Read the model definition and answer for the solid it produces. Units are mm, in the model's axes. Face numbers are marked on the shaded views. A direction names the side the tool comes from. Round coordinates to 2 decimals unless told otherwise and drop trailing zeros. Order: outer loops, then holes, each group sorted by start corner. A loop starts at its lowest first (then second) coordinate and runs counter-clockwise, first axis right, second up. Notation, with made-up numbers: (-29, 65) - (26, 65) arc R24 cw to (26, 95) - close; hole circle Ø10 at (81.5, 83.5). An arc over 180 degrees is marked (long way). Put each result on its own line as item: value. Start each with the question number.
Q1. Each of these flat-tipped pins is pushed along its axis until it touches: pin 1 Ø22 at (x, y) = (8, -12.5) entering from +Z; pin 2 Ø3 at (x, z) = (-8.5, 17.5) entering from -Y; pin 3 Ø2.5 at (y, z) = (26.5, 17.5) entering from +X. Where does it stop, or does it pass through?
Q2. Section C-C on x = 16 is taken. Give the vertices of the cut face in (y, z).
Q3. Find the intervals of material crossed by line 1 along Y through (x, z) = (-8.5, 8.3); line 2 along Y through (x, z) = (16, 1); line 3 along Z through (x, y) = (-19.5, -22), in increasing order. Write a range as from..to.
Q4. Section A-A on y = -32.5 is taken. Give the vertices of the cut face in (x, z).
Q5. Section B-B on z = 18.3 is taken. Give the vertices of the cut face in (x, y).
Q6. Which of the six approach directions +Z, -Z, +X, -X, +Y, -Y give full straight-line access (tool end or side, diameter ignored) to the marked faces 1 and 2?
Q7. Section D-D on z = 5.25 is taken. Give the vertices of the cut face in (x, y).
from build123d import *

# Parameters (mm, degrees)
SKETCH1_W           = 50
SKETCH1_H           = 75
SKETCH1_R           = 1.5
BOSS_EXTRUDE1_DEPTH = 3
SKETCH2_W           = 4
SKETCH2_H           = 9
BOSS_EXTRUDE2_DEPTH = 20
SKETCH3_R           = 1.5
CUT_EXTRUDE2_DEPTH  = 57.216100896
SKETCH4_W           = 5.5
SKETCH4_H           = 75
CUT_EXTRUDE3_DEPTH  = 10


with BuildPart() as part:
    # Sketch1 → Boss-Extrude1 (new body)
    with BuildSketch(Plane.XY):
        Rectangle(SKETCH1_W, SKETCH1_H)
        with Locations((-11, 32.5)):
            Circle(SKETCH1_R, mode=Mode.SUBTRACT)
        with Locations((16, 32.5)):
            Circle(SKETCH1_R, mode=Mode.SUBTRACT)
        with Locations((16, -32.5)):
            Circle(SKETCH1_R, mode=Mode.SUBTRACT)
        with Locations((-11, -32.5)):
            Circle(SKETCH1_R, mode=Mode.SUBTRACT)
    extrude(amount=BOSS_EXTRUDE1_DEPTH)

    # Sketch2 → Boss-Extrude2 (add)
    with BuildSketch(Plane.XY.offset(3)):
        with Locations((-8, 24.8)):
            Rectangle(SKETCH2_W, SKETCH2_H)
    boss_extrude2 = extrude(amount=BOSS_EXTRUDE2_DEPTH)

    # Sketch3 → Cut-Extrude2 (cut, symmetric)
    with BuildSketch(Plane.ZY.offset(10)):
        with Locations((18.3, 24.8)):
            Circle(SKETCH3_R)
        with Locations((8.3, 24.8)):
            Circle(SKETCH3_R)
    cut_extrude2 = extrude(amount=CUT_EXTRUDE2_DEPTH, both=True, mode=Mode.SUBTRACT)

    # Mirror3: Boss-Extrude2, Cut-Extrude2 across plane
    add(boss_extrude2.mirror(Plane.ZX))
    add(cut_extrude2.mirror(Plane.ZX), mode=Mode.SUBTRACT)

    # Sketch4 → Cut-Extrude3 (cut)
    with BuildSketch(Plane.XY.offset(3)):
        with Locations((22.25, 0)):
            Rectangle(SKETCH4_W, SKETCH4_H)
    extrude(amount=-CUT_EXTRUDE3_DEPTH, mode=Mode.SUBTRACT)


solid = part.part
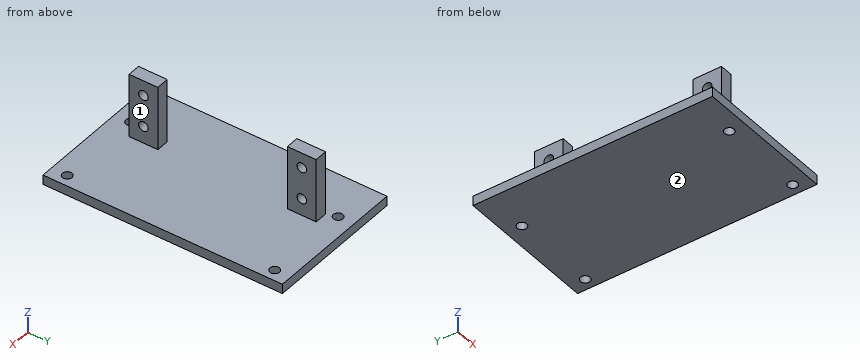
Findings:
1. pin 1: z = 3
1. pin 2: y = -29.3
1. pin 3: x = -6
2. outline: (-37.5, 0) - (-34, 0) - (-34, 3) - (-37.5, 3) - close; (-31, 0) - (31, 0) - (31, 3) - (-31, 3) - close; (34, 0) - (37.5, 0) - (37.5, 3) - (34, 3) - close
3. line 1: -29.3..-26.3, -23.3..-20.3, 20.3..23.3, 26.3..29.3
3. line 2: -37.5..-34, -31..31, 34..37.5
3. line 3: 0..3
4. outline: (-25, 0) - (-12.5, 0) - (-12.5, 3) - (-25, 3) - close; (-9.5, 0) - (14.5, 0) - (14.5, 3) - (-9.5, 3) - close; (17.5, 0) - (19.5, 0) - (19.5, 3) - (17.5, 3) - close
5. outline: (-10, -29.3) - (-6, -29.3) - (-6, -26.3) - (-10, -26.3) - close; (-10, -23.3) - (-6, -23.3) - (-6, -20.3) - (-10, -20.3) - close; (-10, 20.3) - (-6, 20.3) - (-6, 23.3) - (-10, 23.3) - close; (-10, 26.3) - (-6, 26.3) - (-6, 29.3) - (-10, 29.3) - close
6. face 1: +Z, +X, +Y, -Y
6. face 2: -Z, +X, -X, +Y, -Y
7. outline: (-10, -29.3) - (-6, -29.3) - (-6, -20.3) - (-10, -20.3) - close; (-10, 20.3) - (-6, 20.3) - (-6, 29.3) - (-10, 29.3) - close
